Build history of the part. All positions in model axes, mm. Face numbers are marked on the shaded views. A direction names the side the tool comes from. Round coordinates to 2 decimals unless told otherwise and drop trailing zeros. Order: outer loops, then holes, each group sorted by start corner. A loop starts at its lowest first (then second) coordinate and runs counter-clockwise, first axis right, second up. Notation, with made-up numbers: M 2.25,-1 L 21.25,-1 A30 ccw 21.25,30 Z; hole C 42,59.25 d5. An arc over 180 degrees is marked long. One line per question, with ' | ' between items. Start each with the question number.
from build123d import *

# Parameters (mm, degrees)
SKETCH_22_R         = 10
EXTRUDE_12_DEPTH    = 17.5
SKETCH_25_R         = 10
EXTRUDE_13_DEPTH    = 35
SKETCH_26_R         = 5
CUT_EXTRUDE_6_DEPTH = 12


with BuildPart() as part:
    # 草图22 → 凸台-拉伸12 (new, symmetric)
    with BuildSketch(Plane(origin=(0, 0, 0), x_dir=(0, 0, -1), z_dir=(1, 0, 0))):
        Circle(SKETCH_22_R)
    extrude(amount=EXTRUDE_12_DEPTH, both=True)

    # 草图25 → 凸台-拉伸13 (add)
    with BuildSketch(Plane.XY):
        with Locations(Location((0, 0, 0), (0, 0, 90))):
            Circle(SKETCH_25_R)
    extrude(amount=EXTRUDE_13_DEPTH)

    # 草图26 → 切除-拉伸6 (cut)
    with BuildSketch(Plane.XY.offset(35)):
        Circle(SKETCH_26_R)
    extrude(amount=-CUT_EXTRUDE_6_DEPTH, mode=Mode.SUBTRACT)


solid = part.part
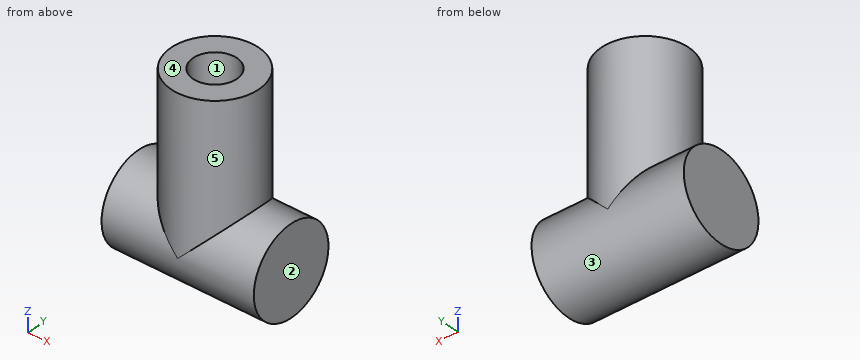
Item 1: Two-plate mould, pull along Y, no slides. Class the marked faces 1, 2 and 3: +Y half, -Y half, draft (parallel to the pull), parting line (faces both ways), or undercut.
Item 2: Cut at C-C on x = 0. Write the cut outline in (y, z), then the cut area to 3 significant figures.
Item 3: Wall check: line 1 along X through (y, z) = (-2, 27.5); line 2 along X through (y, z) = (2.5, 29); line 3 along Y through (x, z) = (-12.5, -3.5). Give the ranges that are in metal, low to high. Write a range as [from, to].
Item 4: Cut at B-B on z = 6. Write the cut outline in (x, y).
Item 5: Cut at D-D on z = 31.5. Write the cut outline in (x, y), then the cut area to 3 significant figures.
Item 6: Cut at A-A on y = 0. Write the cut outline in (x, z), then the cut area to 3 significant figures.
Item 7: Flat gauge pins, fed straight in: pin 1 (1 mm diameter, centred on x = -3.5, y = 1, fed in from +Z); pin 2 (8 mm diameter, centred on x = 0.5, y = 1.5, fed in from +Z); pin 3 (12 mm diameter, centred on x = -7.5, z = 15.5, fed in from +Y); pin 4 (1.5 mm diameter, centred on y = 3.5, z = 15.5, fed in from -X). Where does each tip first touch, or does it go through?
Item 8: Tool access for the marked faces 4 and 5: list every direction of +Z, -Z, +X, -X, +Y, -Y with a clear straight run to the whole face (end or side of a thin tool).
Results found:
1) face 1: undercut | face 2: draft | face 3: parting line
2) outline: M -10,0 A10 ccw 10,0 L 10,35 L 5,35 L 5,23 L -5,23 L -5,35 L -10,35 Z | area: 737 mm^2
3) line 1: x = [-9.8, -4.58], [4.58, 9.8] | line 2: x = [-9.68, -4.33], [4.33, 9.68] | line 3: y = [-9.37, 9.37]
4) outline: M -17.5,-8 L -6,-8 A10 ccw 6,-8 L 17.5,-8 L 17.5,8 L 6,8 A10 ccw -6,8 L -17.5,8 Z
5) outline: C 0,0 d20; hole C 0,0 d10 | area: 236 mm^2
6) outline: M -17.5,-10 L 17.5,-10 L 17.5,10 L 10,10 L 10,35 L 5,35 L 5,23 L -5,23 L -5,35 L -10,35 L -10,10 L -17.5,10 Z | area: 1,080 mm^2
7) pin 1: stops at z = 23 | pin 2: stops at z = 35 | pin 3: stops at y = 9.89 | pin 4: stops at x = -9.61
8) face 4: +Z, +X, -X, +Y, -Y | face 5: +Z
